The listing builds one solid part. Answer for the finished solid, in the listing's coordinates (mm). Face numbers are marked on the shaded views. A direction names the side the tool comes from. Give positions to 0.01 mm unless a question says otherwise; leave off trailing zeros. Order: outer loops, then holes, each group sorted by start corner. A loop starts at its lowest first (then second) coordinate and runs counter-clockwise, first axis right, second up. Notation, with made-up numbers: (10.5, 36) - (16.5, 36) arc R19 ccw to (16.5, 71) - close; hole circle Ø4 at (47, 71). An arc over 180 degrees is marked (long way). Answer as a JSON object with one key per item and string values. Group by question number.
Q1. A cutting plane is placed at B-B, the plane y = 4. Give the vertices of the cut face in (x, z), and give its area (3 significant figures).
Q2. A cutting plane is placed at C-C, the plane x = 0. Give the vertices of the cut face in (y, z), and give its area (3 significant figures).
Q3. The mould has two halves that part along X. Classify the marked faces 1, 2 and 3: released by +X, released by -X, zero draft, split by the parting line, or undercut.
Q4. Consider line 1 (X direction, y = -0.5, z = 0.7); line 2 (Y direction, x = -6, z = 2.65); line 3 (X direction, y = 0.5, z = 3.1). Determine where each line is inside the solid, lowest interval first.
Q5. A cutting plane is placed at A-A, the plane z = 1.55. Give the vertices of the cut face in (x, y), and give its area (3 significant figures).
Q6. For the marked faces 4 and 5, determine the directions among +Z, -Z, +X, -X, +Y, -Y from which every point of the face is accessible in a straight line to the end or side of a thin tool.
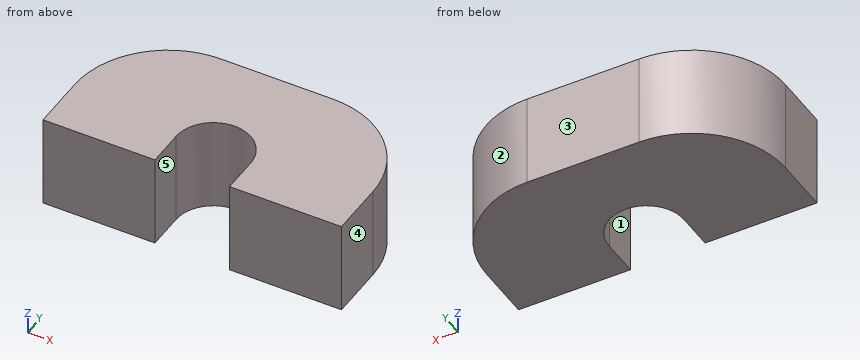
from build123d import *

# Parameters (mm, degrees)
F1_DEPTH = 5


with BuildPart() as f1:
    # F0 (on Top) → F1 (new body)
    with BuildSketch(Plane.XY):
        with BuildLine():
            ThreePointArc((-2, 0), (0, 2), (2, 0))
            Line((2, 0), (2, -2))
            Line((2, -2), (8, -2))
            Line((8, -2), (8, 1))
            ThreePointArc((8, 1), (6.535534, 4.535534), (3, 6))
            Line((3, 6), (-3, 6))
            ThreePointArc((-3, 6), (-6.535534, 4.535534), (-8, 1))
            Line((-8, 1), (-8, -2))
            Line((-8, -2), (-2, -2))
            Line((-2, -2), (-2, 0))
        make_face()
    extrude(amount=F1_DEPTH)


solid = f1.part
Reply:
{
 "1": {"outline": "(-7, 0) - (7, 0) - (7, 5) - (-7, 5) - close", "area": "70.0 mm^2"},
 "2": {"outline": "(2, 0) - (6, 0) - (6, 5) - (2, 5) - close", "area": "20.0 mm^2"},
 "3": {"face 1": "undercut", "face 2": "released by +X", "face 3": "zero draft"},
 "4": {"line 1": "x = -8 to -2, 2 to 8", "line 2": "y = -2 to 5", "line 3": "x = -8 to -1.94, 1.94 to 8"},
 "5": {"outline": "(-8, -2) - (-2, -2) - (-2, 0) arc R2 cw to (2, 0) - (2, -2) - (8, -2) - (8, 1) arc R5 ccw to (3, 6) - (-3, 6) arc R5 ccw to (-8, 1) - close", "area": "103 mm^2"},
 "6": {"face 4": "+Z, -Z, +X, +Y, -Y", "face 5": "+Z, -Z, -Y"}
}
